Verification items for the finished model (mm, model axes). Round coordinates to 2 decimals unless told otherwise and drop trailing zeros. Order: outer loops, then holes, each group sorted by start corner. A loop starts at its lowest first (then second) coordinate and runs counter-clockwise, first axis right, second up. Notation, with made-up numbers: (60.25, 74.25) -> (110.25, 74.25) arc R17 ccw to (110.25, 105.25) -> close; hole circle Ø9 at (72.5, 49). An arc over 180 degrees is marked (long way). Write item = value, one per line. Start each with the question number.
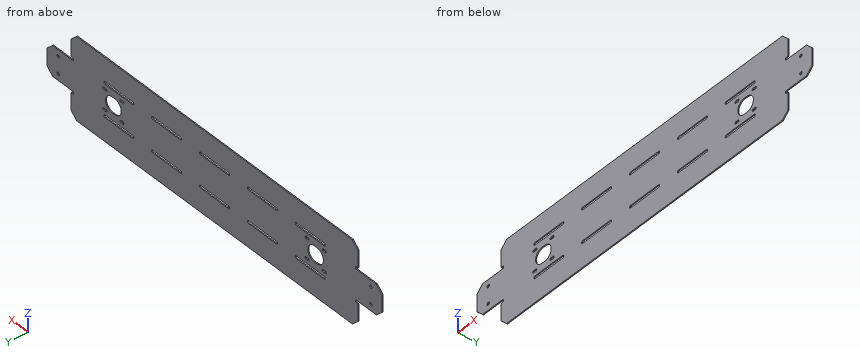
from build123d import *

# Parameters (mm, degrees)
BOSS_EXTRUDE1_DEPTH = 1.5
CUT_EXTRUDE2_DEPTH  = 3
SKETCH4_R           = 2.25
CUT_EXTRUDE3_DEPTH  = 10
CHAMFER3_SIZE       = 10
CHAMFER4_SIZE       = 10


with BuildPart() as part:
    # Sketch1 → Boss-Extrude1 (new body)
    with BuildSketch(Plane(origin=(0, 0, 0), x_dir=(1, 0, 0), z_dir=(0, 1, 0))):
        with BuildLine():
            Line((300, 2), (300, 48))
            Line((300, 48), (275, 48))
            ThreePointArc((275, 48), (273, 50), (275, 52))
            Line((275, 52), (300, 52))
            Line((300, 52), (300, 88))
            Line((300, 88), (43, 88))
            Line((43, 88), (43, 52))
            Line((43, 52), (45.783630632, 52))
            ThreePointArc((45.783630632, 52), (47.783630632, 50), (45.783630632, 48))
            Line((45.783630632, 48), (43, 48))
            Line((43, 48), (0, 48))
            Line((0, 48), (0, 2))
            Line((0, 2), (43, 2))
            Line((43, 2), (45.783630632, 2))
            ThreePointArc((45.783630632, 2), (47.783630632, 0), (45.783630632, -2))
            Line((45.783630632, -2), (43, -2))
            Line((43, -2), (43, -38))
            Line((43, -38), (300, -38))
            Line((300, -38), (300, -2))
            Line((300, -2), (275, -2))
            ThreePointArc((275, -2), (273, 0), (275, 2))
            Line((275, 2), (300, 2))
        make_face()
        with BuildLine():
            Line((103.666666667, 2), (153.666666667, 2))
            ThreePointArc((153.666666667, 2), (155.666666667, 0), (153.666666667, -2))
            Line((153.666666667, -2), (103.666666667, -2))
            ThreePointArc((103.666666667, -2), (101.666666667, 0), (103.666666667, 2))
        make_face(mode=Mode.SUBTRACT)
        with BuildLine():
            Line((189.333333333, 2), (239.333333333, 2))
            ThreePointArc((239.333333333, 2), (241.333333333, 0), (239.333333333, -2))
            Line((239.333333333, -2), (189.333333333, -2))
            ThreePointArc((189.333333333, -2), (187.333333333, 0), (189.333333333, 2))
        make_face(mode=Mode.SUBTRACT)
        with BuildLine():
            Line((189.333333333, 48), (239.333333333, 48))
            ThreePointArc((239.333333333, 48), (241.333333333, 50), (239.333333333, 52))
            Line((239.333333333, 52), (189.333333333, 52))
            ThreePointArc((189.333333333, 52), (187.333333333, 50), (189.333333333, 48))
        make_face(mode=Mode.SUBTRACT)
        with BuildLine():
            Line((103.666666667, 48), (153.666666667, 48))
            ThreePointArc((153.666666667, 48), (155.666666667, 50), (153.666666667, 52))
            Line((153.666666667, 52), (103.666666667, 52))
            ThreePointArc((103.666666667, 52), (101.666666667, 50), (103.666666667, 48))
        make_face(mode=Mode.SUBTRACT)
    extrude(amount=BOSS_EXTRUDE1_DEPTH)

    # Sketch3 → Cut-Extrude2 (cut)
    with BuildSketch(Plane(origin=(0, 1.5, 0), x_dir=(1, 0, 0), z_dir=(0, 1, 0))):
        with BuildLine():
            Line((117, 37), (121, 37))
            ThreePointArc((121, 37), (133, 25), (121, 13))
            Line((121, 13), (117, 13))
            ThreePointArc((117, 13), (105, 25), (117, 37))
        make_face()
        with BuildLine():
            Line((101.5, 11.25), (105.5, 11.25))
            ThreePointArc((105.5, 11.25), (107.25, 9.5), (105.5, 7.75))
            Line((105.5, 7.75), (101.5, 7.75))
            ThreePointArc((101.5, 7.75), (99.75, 9.5), (101.5, 11.25))
        make_face()
        with BuildLine():
            Line((136.5, 7.75), (132.5, 7.75))
            ThreePointArc((132.5, 7.75), (130.75, 9.5), (132.5, 11.25))
            Line((132.5, 11.25), (136.5, 11.25))
            ThreePointArc((136.5, 11.25), (138.25, 9.5), (136.5, 7.75))
        make_face()
        with BuildLine():
            Line((132.5, 42.25), (136.5, 42.25))
            ThreePointArc((136.5, 42.25), (138.25, 40.5), (136.5, 38.75))
            Line((136.5, 38.75), (132.5, 38.75))
            ThreePointArc((132.5, 38.75), (130.75, 40.5), (132.5, 42.25))
        make_face()
        with BuildLine():
            Line((105.5, 38.75), (101.5, 38.75))
            ThreePointArc((101.5, 38.75), (99.75, 40.5), (101.5, 42.25))
            Line((101.5, 42.25), (105.5, 42.25))
            ThreePointArc((105.5, 42.25), (107.25, 40.5), (105.5, 38.75))
        make_face()
    extrude(amount=-CUT_EXTRUDE2_DEPTH, mode=Mode.SUBTRACT)

    # Mirror3: part across plane


with BuildPart() as part_1:
    add(part.part)
    add(part.part.mirror(Plane(origin=(300, 0, 0), x_dir=(0, 0, 1), z_dir=(1, 0, 0))))

    # Sketch4 → Cut-Extrude3 (cut)
    with BuildSketch(Plane(origin=(0, 1.5, 0), x_dir=(1, 0, 0), z_dir=(0, 1, 0))):
        with Locations(Location((20, 38, 0), (0, 0, 270))):
            Circle(SKETCH4_R)
        with Locations(Location((20, 12, 0), (0, 0, 270))):
            Circle(SKETCH4_R)
    cut_extrude3 = extrude(amount=-CUT_EXTRUDE3_DEPTH, mode=Mode.SUBTRACT)

    # Mirror4: Cut-Extrude3 across plane
    add(cut_extrude3.mirror(Plane(origin=(300, 0, 0), x_dir=(0, 0, 1), z_dir=(1, 0, 0))), mode=Mode.SUBTRACT)

    # Chamfer3
    chamfer3_edges = [part_1.edges().sort_by_distance(p)[0] for p in [
        (43, 0.75, 38),
        (0, 0.75, -2),
        (0, 0.75, -48),
        (43, 0.75, -88),
    ]]
    chamfer(chamfer3_edges, length=CHAMFER3_SIZE)

    # Chamfer4
    chamfer4_edges = [part_1.edges().sort_by_distance(p)[0] for p in [
        (557, 0.75, -88),
        (600, 0.75, -48),
        (600, 0.75, -2),
        (557, 0.75, 38),
    ]]
    chamfer(chamfer4_edges, length=CHAMFER4_SIZE)


solid = part_1.part
(1) Cross-section at B-B (y = 0.3). Give the number of separate pieces and of enclosed holes in the cut face, and give its area (3 significant figures).
(2) Depth check by flat-ended pin: pin 1 (0.8 mm diameter, centred on y = 1, z = -61.5, fed in from +X). Enter the tip coordinate at first touch or a pass-through.
(3) Cross-section at A-A (x = 225). Enter the section's corners in (y, z).
(4) Scan lines: line 1 along X through (y, z) = (1.1, -38); line 2 along Z through (x, y) = (580, 0.8); line 3 along Z through (x, y) = (310.5, 0.75). Record each from-to range of solid material in increasing order. Write a range as from..to.
Outcome:
q1.separate_pieces = 1
q1.enclosed_holes = 24
q1.area = 64,800 mm^2
q2.pin_1 = 557
q3.outline = (0, -88) -> (1.5, -88) -> (1.5, -52) -> (0, -52) -> close; (0, -48) -> (1.5, -48) -> (1.5, -2) -> (0, -2) -> close; (0, 2) -> (1.5, 2) -> (1.5, 38) -> (0, 38) -> close
q4.line_1 = 0..17.75, 22.25..577.75, 582.25..600
q4.line_2 = -48..-40.25, -35.75..-14.25, -9.75..-2
q4.line_3 = -88..-52, -48..-2, 2..38
